Design review of the part built by this model. Coordinates are the model's own, in mm. A direction names the side the tool comes from. Coordinates: 2 decimals unless noted, no trailing zeros. Write each loop counter-clockwise with the first axis right and the second up, starting at its lowest first coordinate (ties: lowest second). Pieces come first, ordered by that corner, then holes. Notation, with made-up numbers: (21, -16) - (31, -16) arc R25 ccw to (31, 10) - close; hole circle Ø6 at (87, 66.25). An arc over 180 degrees is marked (long way). Answer as a JSON object with one key per item and string values.
```python
from build123d import *

# Parameters (mm, degrees)
SKETCH1_W           = 1500
SKETCH1_H           = 400
BOSS_EXTRUDE1_DEPTH = 5
SKETCH3_W           = 1494
SKETCH3_H           = 394
BOSS_EXTRUDE3_DEPTH = 5
SKETCH4_W           = 1488
SKETCH4_H           = 388
BOSS_EXTRUDE4_DEPTH = 5
SKETCH6_W           = 1386
SKETCH6_H           = 286
CUT_EXTRUDE1_DEPTH  = 1
SKETCH7_W           = 1400
SKETCH7_H           = 370
BOSS_EXTRUDE5_DEPTH = 750
CUT_EXTRUDE2_DEPTH  = 320
CUT_EXTRUDE3_DEPTH  = 30.65
CUT_EXTRUDE4_DEPTH  = 30.65
CUT_EXTRUDE6_DEPTH  = 33.56


with BuildPart() as part:
    # Sketch1 → Boss-Extrude1 (new body)
    with BuildSketch(Plane(origin=(0, 0, 0), x_dir=(1, 0, 0), z_dir=(0, 1, 0))):
        Rectangle(SKETCH1_W, SKETCH1_H)
    extrude(amount=BOSS_EXTRUDE1_DEPTH)

    # Sketch3 → Boss-Extrude3 (add)
    with BuildSketch(Plane(origin=(0, 5, 0), x_dir=(1, 0, 0), z_dir=(0, 1, 0))):
        Rectangle(SKETCH3_W, SKETCH3_H)
    extrude(amount=BOSS_EXTRUDE3_DEPTH)

    # Sketch4 → Boss-Extrude4 (add)
    with BuildSketch(Plane(origin=(0, 10, 0), x_dir=(1, 0, 0), z_dir=(0, 1, 0))):
        Rectangle(SKETCH4_W, SKETCH4_H)
    extrude(amount=BOSS_EXTRUDE4_DEPTH)

    # Sketch6 → Cut-Extrude1 (cut)
    with BuildSketch(Plane(origin=(0, 15, 0), x_dir=(1, 0, 0), z_dir=(0, 1, 0))):
        Polygon((744, 194), (743, 194), (693, 144), (-693, 144), (-743, 194), (-744, 194), (-744, 193), (-694, 143), (-694, -143), (-744, -193), (-744, -194), (-743, -194), (-693, -144), (693, -144), (743, -194), (744, -194), (744, -193), (694, -143), (694, 143), (744, 193), align=None)
        Rectangle(SKETCH6_W, SKETCH6_H, mode=Mode.SUBTRACT)
    extrude(amount=-CUT_EXTRUDE1_DEPTH, mode=Mode.SUBTRACT)

    # Sketch7 → Boss-Extrude5 (add)
    with BuildSketch(Plane.XZ):
        Rectangle(SKETCH7_W, SKETCH7_H)
    extrude(amount=BOSS_EXTRUDE5_DEPTH)

    # Sketch8 → Cut-Extrude2 (cut)
    with BuildSketch(Plane.XY.offset(185)):
        Polygon((-625, -250), (-275, -250), (-275, -470), (-295, -470), (-295, -490), (-275, -490), (-275, -690), (-625, -690), (-625, -490), (-605, -490), (-605, -470), (-625, -470), align=None)
        Polygon((-175, -250), (175, -250), (175, -470), (155, -470), (155, -490), (175, -490), (175, -690), (-175, -690), (-175, -490), (-155, -490), (-155, -470), (-175, -470), align=None)
        Polygon((275, -250), (625, -250), (625, -470), (605, -470), (605, -490), (625, -490), (625, -690), (275, -690), (275, -490), (295, -490), (295, -470), (275, -470), align=None)
        Polygon((-625, -175), (-275, -175), (-275, -122.5), (-295, -122.5), (-295, -102.5), (-275, -102.5), (-275, -50), (-625, -50), (-625, -102.5), (-605, -102.5), (-605, -122.5), (-625, -122.5), align=None)
        Polygon((-175, -175), (175, -175), (175, -122.5), (155, -122.5), (155, -102.5), (175, -102.5), (175, -50), (-175, -50), (-175, -102.5), (-155, -102.5), (-155, -122.5), (-175, -122.5), align=None)
        Polygon((275, -102.5), (275, -50), (625, -50), (625, -102.5), (605, -102.5), (605, -122.5), (625, -122.5), (625, -175), (275, -175), (275, -122.5), (295, -122.5), (295, -102.5), align=None)
    extrude(amount=-CUT_EXTRUDE2_DEPTH, mode=Mode.SUBTRACT)

    # Sketch9 → Cut-Extrude3 (cut)
    with BuildSketch(Plane(origin=(-625, 0, 0), x_dir=(0, 0, -1), z_dir=(1, 0, 0))):
        with BuildLine():
            Line((-150, -270), (-150, -360))
            ThreePointArc((-150, -360), (-165, -370), (-180, -360))
            Line((-180, -360), (-180, -320))
            Line((-180, -320), (-185, -320))
            Line((-185, -320), (-185, -270))
            Line((-185, -270), (-150, -270))
        make_face()
        with BuildLine():
            Line((-150, -570), (-150, -660))
            ThreePointArc((-150, -660), (-165, -670), (-180, -660))
            Line((-180, -660), (-180, -620))
            Line((-180, -620), (-185, -620))
            Line((-185, -620), (-185, -570))
            Line((-185, -570), (-150, -570))
        make_face()
    extrude(amount=-CUT_EXTRUDE3_DEPTH, mode=Mode.SUBTRACT)

    # Sketch10 → Cut-Extrude4 (cut)
    with BuildSketch(Plane(origin=(-175, 0, 0), x_dir=(0, 0, -1), z_dir=(1, 0, 0))):
        with BuildLine():
            Line((-150, -270), (-150, -360))
            ThreePointArc((-150, -360), (-165, -370), (-180, -360))
            Line((-180, -360), (-180, -320))
            Line((-180, -320), (-185, -320))
            Line((-185, -320), (-185, -270))
            Line((-185, -270), (-150, -270))
        make_face()
        with BuildLine():
            Line((-150, -570), (-150, -660))
            ThreePointArc((-150, -660), (-165, -670), (-180, -660))
            Line((-180, -660), (-180, -620))
            Line((-180, -620), (-185, -620))
            Line((-185, -620), (-185, -570))
            Line((-185, -570), (-150, -570))
        make_face()
    extrude(amount=-CUT_EXTRUDE4_DEPTH, mode=Mode.SUBTRACT)

    # Sketch12 → Cut-Extrude6 (cut)
    with BuildSketch(Plane.ZY.offset(-625)):
        with BuildLine():
            Line((150, -270), (150, -360))
            ThreePointArc((150, -360), (165, -370), (180, -360))
            Line((180, -360), (180, -320))
            Line((180, -320), (185, -320))
            Line((185, -320), (185, -270))
            Line((185, -270), (150, -270))
        make_face()
        with BuildLine():
            Line((150, -570), (150, -660))
            ThreePointArc((150, -660), (165, -670), (180, -660))
            Line((180, -660), (180, -620))
            Line((180, -620), (185, -620))
            Line((185, -620), (185, -570))
            Line((185, -570), (150, -570))
        make_face()
    extrude(amount=-CUT_EXTRUDE6_DEPTH, mode=Mode.SUBTRACT)


solid = part.part
```
(1) The part is to be moulded in two halves that separate along X. For faces 4 (the face through (175, -358, 27)), 5 (the face through (642, -370, 165)), 6 (the face through (-700, -370, -3)), say which applies: pulls with the +X half, pulls with the -X half, needs draft (parallel to the pull), parting line crosses it, or undercut.
Solved:
{"face 4": "undercut", "face 5": "undercut", "face 6": "pulls with the -X half"}
(2) To check wall thickness, follow line 1 (X direction, y = -504.5, z = -47.5); line 2 (Y direction, x = -485.5, z = 141); line 3 (X direction, y = -332.5, z = 155). State the ranges of each line that lie inside material, in increasing order. Write a range as from..to.
Solved:
{"line 1": "x = -700..-625, -275..-175, 175..275, 625..700", "line 2": "y = -750..-690, -250..-175, -50..15", "line 3": "x = -700..-655.65, -275..-205.65, 175..275, 658.56..700"}
(3) Take a section at A-A, the plane x = 206.5. Write out the cut boundary in (y, z).
Solved:
{"outline": "(-750, -185) - (0, -185) - (0, -200) - (5, -200) - (5, -197) - (10, -197) - (10, -194) - (15, -194) - (15, -144) - (14, -144) - (14, -143) - (15, -143) - (15, 143) - (14, 143) - (14, 144) - (15, 144) - (15, 194) - (10, 194) - (10, 197) - (5, 197) - (5, 200) - (0, 200) - (0, 185) - (-750, 185) - close"}
(4) Take a section at B-B, the plane y = -75. Write out the cut boundary in (x, z), and give its area (3 significant figures).
Solved:
{"outline": "(-700, -185) - (700, -185) - (700, 185) - (625, 185) - (625, -135) - (275, -135) - (275, 185) - (175, 185) - (175, -135) - (-175, -135) - (-175, 185) - (-275, 185) - (-275, -135) - (-625, -135) - (-625, 185) - (-700, 185) - close", "area": "182,000 mm^2"}
(5) Tool access review of faces 1 (the face through (-640, -614, 150)), 2 (the face through (452, -690, 27)), 3 (the face through (-719.4, 14.5, -168.4)): name each direction out of +Z, -Z, +X, -X, +Y, -Y from which nothing blocks a thin tool from reaching the whole face with its end or side.
Solved:
{"face 1": "none", "face 2": "+Z", "face 3": "+Y"}
(6) Take a section at D-D, the plane y = -301. Write out the cut boundary in (x, z), and give its area (3 significant figures).
Solved:
{"outline": "(-700, -185) - (700, -185) - (700, 185) - (658.56, 185) - (658.56, 150) - (625, 150) - (625, -135) - (275, -135) - (275, 185) - (175, 185) - (175, -135) - (-175, -135) - (-175, 150) - (-205.65, 150) - (-205.65, 185) - (-275, 185) - (-275, -135) - (-625, -135) - (-625, 150) - (-655.65, 150) - (-655.65, 185) - (-700, 185) - close", "area": "179,000 mm^2"}
(7) Take a section at C-C, the plane z = 33. Give the number of separate pieces and of enclosed holes in the cut face, and give its area (3 significant figures).
Solved:
{"separate pieces": "1", "enclosed holes": "6", "area": "484,000 mm^2"}
(8) For pin 1 (5 mm diameter, centred on y = -334.5, z = -68, fed in from +X); pin 2 (15.5 mm diameter, centred on x = -641.5, y = -326, fed in from +Z); pin 3 (22 mm diameter, centred on y = -478, z = 4, fed in from -X), all flat-tipped, find the tip position at first contact; note any pin that passes through.
Solved:
{"pin 1": "stops at x = 700", "pin 2": "stops at z = 185", "pin 3": "stops at x = -700"}
